Check sheet for the drawn part. Datum: minimum x, y, z corner. Units: mm. Give positions to 0.01 mm unless a question says otherwise; leave off trailing zeros. Order: outer loops, then holes, each group sorted by start corner. A loop starts at its lowest first (then second) coordinate and runs counter-clockwise, first axis right, second up.
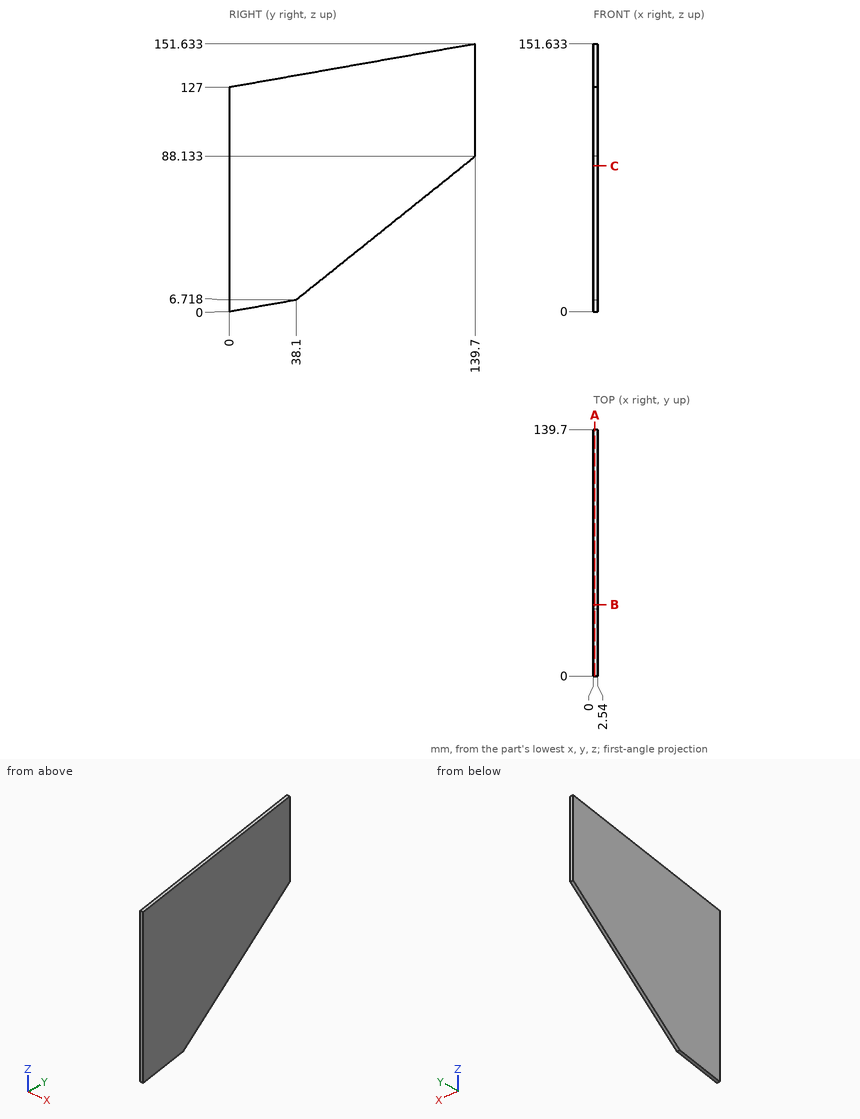
Q1. Sectioned sample at A-A, the plane x = 0.8. Record the cut outline in (y, z).
Q2. Sectioned sample at B-B, the plane y = 40.5. Record the cut outline in (x, z), plus the area to 3 significant figures.
Q3. Sectioned sample at C-C, the plane z = 82.5. Record the cut outline in (x, y).
Q4. Material ranges on line 1 (Z direction, x = 0.4, y = 72) (1 decimal); line 2 (Z direction, x = 0.6, y = 7); line 3 (Y direction, x = 1.05, z = 16), recorded low to high.
Filled in:
1. outline: (0, 0) - (38.1, 6.72) - (139.7, 88.13) - (139.7, 151.63) - (0, 127) - close
2. outline: (0, 8.64) - (2.54, 8.64) - (2.54, 134.14) - (0, 134.14) - close
2. area: 319 mm2
3. outline: (0, 0) - (2.54, 0) - (2.54, 132.67) - (0, 132.67) - close
4. line 1: z = 33.9 to 139.7
4. line 2: z = 1.23 to 128.23
4. line 3: y = 0 to 49.68
